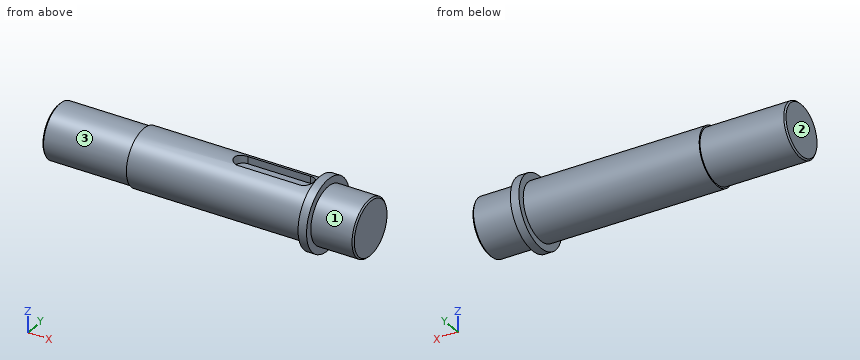
```python
from build123d import *

# Parameters (mm, degrees)
CUT_EXTRUDE_1_DEPTH = 3
CHAMFER_1_SIZE      = 0.5
CHAMFER_2_SIZE      = 0.5


with BuildPart() as part:
    # 草图1 → 旋转1 (revolve)
    with BuildSketch(Plane.XY):
        Polygon((0, 0), (0, 9.5), (30, 9.5), (30, 10), (92, 10), (92, 12.5), (95, 12.5), (95, 10), (110, 10), (110, 0), align=None)
    revolve(axis=Axis((-40.465116279, 0, 0), (1, 0, 0)))

    # 草图3 → 切除-拉伸1 (cut)
    with BuildSketch(Plane.XY.offset(10)):
        with BuildLine():
            Line((65, 3), (87, 3))
            ThreePointArc((87, 3), (90, 0), (87, -3))
            Line((87, -3), (65, -3))
            ThreePointArc((65, -3), (62, 0), (65, 3))
        make_face()
    extrude(amount=-CUT_EXTRUDE_1_DEPTH, mode=Mode.SUBTRACT)

    # 倒角1
    chamfer_1_edges = [part.edges().sort_by_distance(p)[0] for p in [
        (0, -9.5, 0),
    ]]
    chamfer(chamfer_1_edges, length=CHAMFER_1_SIZE)

    # 倒角2
    chamfer_2_edges = [part.edges().sort_by_distance(p)[0] for p in [
        (110, -10, 0),
    ]]
    chamfer(chamfer_2_edges, length=CHAMFER_2_SIZE)


solid = part.part
```
The model under review builds one solid part; all positions refer to its coordinate system, in mm. Face numbers are marked on the shaded views. A direction names the side the tool comes from. Round coordinates to 2 decimals unless told otherwise and drop trailing zeros. Loops run counter-clockwise (first coordinate to the right, second up) from the corner with the lowest first, then second, coordinate; pieces in that order, holes last. Notation, with made-up numbers: M 46,52.5 L 66,52.5 A34 ccw 66,90.5 Z; hole C 7,-38 d4. An arc over 180 degrees is marked long. Write item = value, one per line.
Item 1: Take a section at A-A on z = 0. Write out the cut boundary in (x, y), then the cut area to 3 significant figures.
Return value:
outline = M 0,-9 L 0.5,-9.5 L 30,-9.5 L 30,-10 L 92,-10 L 92,-12.5 L 95,-12.5 L 95,-10 L 109.5,-10 L 110,-9.5 L 110,9.5 L 109.5,10 L 95,10 L 95,12.5 L 92,12.5 L 92,10 L 30,10 L 30,9.5 L 0.5,9.5 L 0,9 Z
area = 2,180 mm2
Item 2: Machinability: for the marked faces 1, 2 and 3, which of the approach directions +Z, -Z, +X, -X, +Y, -Y give a long, thin tool a straight path to every point of the face, cutting with its end or side? Answer none if there is none.
Return value:
face_1 = +X
face_2 = +Z, -Z, -X, +Y, -Y
face_3 = -X
Item 3: Take a section at B-B on x = 56. Write out the cut boundary in (y, z), then the cut area to 3 significant figures.
Return value:
outline = C 0,0 d20
area = 314 mm2
Item 4: Take a section at D-D on x = 72.5. Write out the cut boundary in (y, z).
Return value:
outline = M -3,7 L -3,9.54 A10 ccw long 3,9.54 L 3,7 Z
Item 5: Insertion check: P1, Ø0.8, axis at x = 78.5, z = 8.5, coming from the -Y side; P2, Ø4, axis at x = 49, z = 4, coming from the +Y side; P3, Ø1.5, axis at x = 99, y = -1, coming from the -Z side. Each pin has a flat end and moves straight along its axis. Give the tip position at first contact, or say it passes through.
Return value:
P1 = -5.86
P2 = 9.8
P3 = -10
Item 6: Take a section at C-C on x = 18.5. Write out the cut boundary in (y, z), then the cut area to 3 significant figures.
Return value:
outline = C 0,0 d19
area = 284 mm2
Item 7: For line 1 (Z direction, x = 69, y = -0.25); line 2 (X direction, y = -2, z = 9); line 3 (X direction, y = -10.75, z = -3.5), list the stretches that pass through material, from the lowest coordinate up. Write a range as [from, to].
Return value:
line_1 = [-10, 7]
line_2 = [0.22, 62.76], [89.24, 110]
line_3 = [92, 95]
